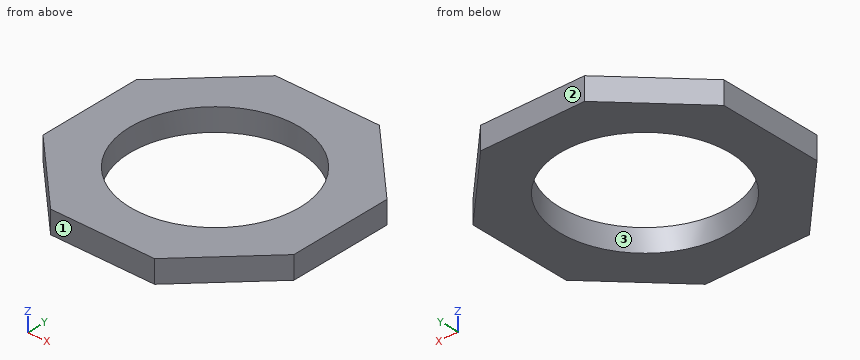
Autodesk Inventor part; units mm, degrees
ref_plane "YZ Plane" through (0, 0, 0) normal (1, 0, 0) x (0, 1, 0)
ref_plane "XZ Plane" through (0, 0, 0) normal (0, 1, 0) x (-1, 0, 0)
ref_plane "XY Plane" through (0, 0, 0) normal (0, 0, 1) x (1, 0, 0)
sketch "Skizze2" plane through (0, 0, 0) normal (0, 0, 1) x (1, 0, 0)
  circle A0 centre (0, 0) radius 67.5
  line L0 (-41.4214, 100) -> (41.4214, 100)
  line L1 (41.4214, 100) -> (100, 41.4214)
  line L2 (100, 41.4214) -> (100, -41.4214)
  line L3 (100, -41.4214) -> (41.4214, -100)
  line L4 (41.4214, -100) -> (-41.4214, -100)
  line L5 (-41.4214, -100) -> (-100, -41.4214)
  line L6 (-100, -41.4214) -> (-100, 41.4214)
  line L7 (-100, 41.4214) -> (-41.4214, 100)
  dimension "d7" = 135
  dimension "d11" = 200
extrude "Extrusion2" add sketch "Skizze2" along normal blind 18
equation "\"kg_thickness\" = 4.9"
equation "\"ht_thickness\" = 1.9"
equation "\"case_thickness\" = 18"
equation "\"inner_thickness\" = 15"
equation "\"gap_fit\" = 0.1"
equation "\"gap_slide\" = 0.2"
equation "\"gap_air\" = 1"
equation "\"bore_diameter\" = 73"
equation "\"mdf_thickness\" = 6"
equation "\"tape_width\" = 15"
equation "\"tape_thickness\" = 3"
equation "\"inner_depth\" = 255"
properties part number "Korpus_Motor_18mm"
Build history of the part. All positions in model axes, mm. Face numbers are marked on the shaded views. Coordinates: 2 decimals unless noted, no trailing zeros. Order: outer loops, then holes, each group sorted by start corner. A loop starts at its lowest first (then second) coordinate and runs counter-clockwise, first axis right, second up. Notation, with made-up numbers: (-1, 83.5) -> (28, 83.5) arc R30 cw to (28, 116.5) -> close; hole circle Ø4 at (30.5, 9). An arc over 180 degrees is marked (long way). Answer in a Markdown table with one row per item. Add a question column.
Q1. Band-saw the part on A-A, the plane x = 0. List the corners of the cut face in (y, z), then the cut area to 3 significant figures.
Q2. Band-saw the part on B-B, the plane z = 15. List the corners of the cut face in (x, y), then the cut area to 3 significant figures.
Q3. Drop flat-ended pins along their axis: pin 1 (4 mm diameter, centred on y = 70.5, z = 13, fed in from -X); pin 2 (1 mm diameter, centred on y = -77, z = 5.5, fed in from -X); pin 3 (1 mm diameter, centred on x = -51.5, z = 8.5, fed in from +Y). Give the stop position or say it passes through.
Q4. Mould opens along Y. For the marked faces 1, 2 and 3 say: +Y half, -Y half, draft (parallel to the pull), parting line (faces both ways), or undercut.
Q5. Band-saw the part on D-D, the plane y = -71.5. List the corners of the cut face in (x, z).
Q6. Wall check: line 1 along Y through (x, z) = (0, 10.75); line 2 along Y through (x, z) = (47, 12); line 3 along X through (y, z) = (-10, 11.5). Give the ranges that are in metal, low to high. Write a range as [from, to].
Answers follow:
| question | item | result |
|---|---|---|
| 1 | outline | (-100, 0) -> (-67.5, 0) -> (-67.5, 18) -> (-100, 18) -> close; (67.5, 0) -> (100, 0) -> (100, 18) -> (67.5, 18) -> close |
| 1 | area | 1,170 mm^2 |
| 2 | outline | (-100, -41.42) -> (-41.42, -100) -> (41.42, -100) -> (100, -41.42) -> (100, 41.42) -> (41.42, 100) -> (-41.42, 100) -> (-100, 41.42) -> close; hole circle Ø135 at (0, 0) |
| 2 | area | 18,800 mm^2 |
| 3 | pin 1 | x = -72.92 |
| 3 | pin 2 | x = -64.92 |
| 3 | pin 3 | y = 90.42 |
| 4 | face 1 | -Y half |
| 4 | face 2 | +Y half |
| 4 | face 3 | undercut |
| 5 | outline | (-69.92, 0) -> (69.92, 0) -> (69.92, 18) -> (-69.92, 18) -> close |
| 6 | line 1 | [-100, -67.5], [67.5, 100] |
| 6 | line 2 | [-94.42, -48.45], [48.45, 94.42] |
| 6 | line 3 | [-100, -66.76], [66.76, 100] |
